from build123d import *

# Parameters (mm, degrees)
ESBO_O1_W                  = 30
ESBO_O1_H                  = 12
RESSALTO_EXTRUS_O1_DEPTH   = 5
CORTE_EXTRUS_O1_DEPTH      = 20.849433241
CORTE_EXTRUS_O1_DEPTH_BACK = 20.849433241
ESBO_O3_R                  = 1.75
CORTE_EXTRUS_O2_DEPTH      = 20
ESBO_O4_R                  = 1.75
CORTE_EXTRUS_O3_DEPTH      = 4
CORTE_EXTRUS_O4_DEPTH      = 20.849433241
CORTE_EXTRUS_O4_DEPTH_BACK = 20.849433241
CHANFRO2_SIZE              = 0.6


with BuildPart() as part:
    # Esboço1 → Ressalto-extrusão1 (new, symmetric)
    with BuildSketch(Plane.XY):
        Rectangle(ESBO_O1_W, ESBO_O1_H)
    extrude(amount=RESSALTO_EXTRUS_O1_DEPTH, both=True)

    # Esboço2 → Corte-extrusão1 (cut, two sides: drawn at the far end of the back side and taken through both)
    with BuildSketch(Plane(origin=(0, 6, 0), x_dir=(1, 0, 0), z_dir=(0, 1, 0)).offset(-CORTE_EXTRUS_O1_DEPTH_BACK)):
        with BuildLine():
            Line((-7.5, 64.244289009), (-7.5, 5))
            ThreePointArc((-7.5, 5), (0, -2.5), (7.5, 5))
            Line((7.5, 5), (7.5, 64.244289009))
            Line((7.5, 64.244289009), (7.5, 182.732867027))
            Line((7.5, 182.732867027), (-7.5, 182.732867027))
            Line((-7.5, 182.732867027), (-7.5, 64.244289009))
        make_face()
    extrude(amount=CORTE_EXTRUS_O1_DEPTH + CORTE_EXTRUS_O1_DEPTH_BACK, mode=Mode.SUBTRACT)

    # Esboço3 → Corte-extrusão2 (cut, through all)
    with BuildSketch(Plane.XY.offset(5)):
        with Locations((11.35, 0)):
            Circle(ESBO_O3_R)
    corte_extrus_o2 = extrude(amount=-CORTE_EXTRUS_O2_DEPTH, mode=Mode.SUBTRACT)

    # Espelhar1: Corte-extrusão2 across plane
    add(corte_extrus_o2.mirror(Plane(origin=(0, 0, 0), x_dir=(0, 0, 1), z_dir=(1, 0, 0))), mode=Mode.SUBTRACT)

    # Esboço4 → Corte-extrusão3 (cut)
    # profile 1 of 2: a face of its own
    with BuildSketch(Plane.XY.offset(5)):
        Polygon((-15, -6), (-8.5, -1.645448267), (-11.35, -3.290896534), (-14.2, -1.645448267), (-14.2, 1.645448267), (-11.35, 3.290896534), (-8.5, 1.645448267), (-15, 6), align=None)
    # profile 2 of 2: a face of its own
    with BuildSketch(Plane.XY.offset(5)):
        Polygon((-11.35, -3.290896534), (-8.5, -1.645448267), (-8.5, 1.645448267), (-11.35, 3.290896534), (-14.2, 1.645448267), (-14.2, -1.645448267), align=None)
        with Locations((-11.35, 0)):
            Circle(ESBO_O4_R, mode=Mode.SUBTRACT)
    corte_extrus_o3 = extrude(amount=-CORTE_EXTRUS_O3_DEPTH, mode=Mode.SUBTRACT)

    # Espelhar2: Corte-extrusão3 across plane
    add(corte_extrus_o3.mirror(Plane(origin=(0, 0, 0), x_dir=(0, 0, 1), z_dir=(1, 0, 0))), mode=Mode.SUBTRACT)

    # Esboço5 → Corte-extrusão4 (cut, two sides: drawn at the far end of the back side and taken through both)
    with BuildSketch(Plane.XZ.offset(6).offset(-CORTE_EXTRUS_O4_DEPTH_BACK)):
        with BuildLine():
            Line((-76.735854523, -34.44642365), (-15, 1))
            ThreePointArc((-15, 1), (0, 5), (15, 1))
            Line((15, 1), (76.735854523, -34.44642365))
            Line((76.735854523, -34.44642365), (76.735854523, 107.930044677))
            Line((76.735854523, 107.930044677), (-76.735854523, 107.930044677))
            Line((-76.735854523, 107.930044677), (-76.735854523, -34.44642365))
        make_face()
    extrude(amount=CORTE_EXTRUS_O4_DEPTH + CORTE_EXTRUS_O4_DEPTH_BACK, mode=Mode.SUBTRACT)

    # Chanfro2
    # the kernel refuses this chamfer: 0.6 mm, written as the material it takes off along each edge
    with BuildSketch(Plane(origin=(-15, 6, -6.543009793), x_dir=(0.9996219169112968, 0.027495876610585904, 0), z_dir=(0, 0, 1)), Plane(origin=(15, 6, 2.543009793), x_dir=(-0.9996219169112968, 0.027495876610585824, 0), z_dir=(0, 0, -1))) as chanfro2_piece_1:
        Polygon((CHANFRO2_SIZE * 0.999621916911, -CHANFRO2_SIZE * 0.0274958766106), (-CHANFRO2_SIZE * 0.0274958766106, -CHANFRO2_SIZE * 0.999621916911), (0, 0), align=None)
    extrude(amount=9.086019586, mode=Mode.SUBTRACT)
    with BuildSketch(Plane(origin=(-16.543009793, 6, -5), x_dir=(0, 0.027495876610585942, 0.9996219169112968), z_dir=(1, 0, 0)), Plane(origin=(5.956990207, 6, -5), x_dir=(0, 0.027495876610585942, 0.9996219169112968), z_dir=(1, 0, 0)), Plane(origin=(16.543009793, -6, -5), x_dir=(0, -0.027495876610585942, 0.9996219169112968), z_dir=(-1, 0, 0)), Plane(origin=(-5.956990207, -6, -5), x_dir=(0, -0.027495876610585942, 0.9996219169112968), z_dir=(-1, 0, 0))) as chanfro2_piece_2:
        Polygon((CHANFRO2_SIZE * 0.999621916911, CHANFRO2_SIZE * 0.0274958766106), (-CHANFRO2_SIZE * 0.0274958766106, CHANFRO2_SIZE * 0.999621916911), (0, 0), align=None)
    extrude(amount=10.586019586, mode=Mode.SUBTRACT)
    with BuildSketch(Plane(origin=(0, 6, -5), x_dir=(0.9788435281484443, 0, -0.20461023288659222), z_dir=(-0.20461023288659222, 0, -0.9788435281484443))) as chanfro2_piece_3:
        Polygon((7.5 + CHANFRO2_SIZE, 0), (7.5, CHANFRO2_SIZE), (7.5, 0), align=None)
    revolve(axis=Axis((0, 6, -5), (0, -1, 0)), revolution_arc=203.613366819, mode=Mode.SUBTRACT)
    with BuildSketch(Plane(origin=(0, 6, -25.125), x_dir=(-0.5416797070080789, 0, 0.8405849719187476), z_dir=(-0.8405849719187476, 0, -0.5416797070080789))) as chanfro2_piece_4:
        Polygon((30.125 - CHANFRO2_SIZE, 0), (30.125, -CHANFRO2_SIZE), (30.125, 0), align=None)
    revolve(axis=Axis((0, 6, -25.125), (0, 1, 0)), revolution_arc=65.596114289, mode=Mode.SUBTRACT)
    with BuildSketch(Plane(origin=(0, -6, -5), x_dir=(0.9788435281484443, 0, -0.20461023288659222), z_dir=(-0.20461023288659222, 0, -0.9788435281484443))) as chanfro2_piece_5:
        Polygon((7.5 + CHANFRO2_SIZE, 0), (7.5, -CHANFRO2_SIZE), (7.5, 0), align=None)
    revolve(axis=Axis((0, -6, -5), (0, -1, 0)), revolution_arc=203.613366819, mode=Mode.SUBTRACT)
    with BuildSketch(Plane(origin=(-15, -6, -6.543009793), x_dir=(0.9996219169112968, -0.027495876610585824, 0), z_dir=(0, 0, 1)), Plane(origin=(15, -6, 2.543009793), x_dir=(-0.9996219169112968, -0.027495876610585904, 0), z_dir=(0, 0, -1))) as chanfro2_piece_6:
        Polygon((CHANFRO2_SIZE * 0.999621916911, CHANFRO2_SIZE * 0.0274958766106), (-CHANFRO2_SIZE * 0.0274958766106, CHANFRO2_SIZE * 0.999621916911), (0, 0), align=None)
    extrude(amount=9.086019586, mode=Mode.SUBTRACT)
    with BuildSketch(Plane(origin=(0, -6, -25.125), x_dir=(-0.5416797070080789, 0, 0.8405849719187476), z_dir=(-0.8405849719187476, 0, -0.5416797070080789))) as chanfro2_piece_7:
        Polygon((30.125, CHANFRO2_SIZE), (30.125 - CHANFRO2_SIZE, 0), (30.125, 0), align=None)
    revolve(axis=Axis((0, -6, -25.125), (0, 1, 0)), revolution_arc=65.596114289, mode=Mode.SUBTRACT)


solid = part.part
Here's how the part is built. I have some questions about the finished solid (model axes, mm). A direction names the side the tool comes from. Coordinates: 2 decimals unless noted, no trailing zeros. Loops run counter-clockwise (first coordinate to the right, second up) from the corner with the lowest first, then second, coordinate; pieces in that order, holes last. Notation, with made-up numbers: (26, 30.25) -> (30, 30.25) arc R34 cw to (30, 66.25) -> close; hole circle Ø8 at (26.5, 25.5). An arc over 180 degrees is marked (long way). Use one line per item in the form item = value. Start each with the question number.
(1) If we section it at B-B (x = 0): Please give me the cut outline in (y, z).
(2) If we section it at D-D (y = 2.75): Please give me the cut outline in (x, z) (3 decimals), then the cut area to 3 significant figures.
(3) We'd pull the mould along Y, two halves only. Please class faces 1 (the face through (-8.5, 0, 2)), 2 (the face through (-0.2, -5.8, 4.6)), 3 (the face through (0, 6, 4)): pulls with the +Y half, pulls with the -Y half, needs draft (parallel to the pull), parting line crosses it, or undercut.
(4) If we section it at C-C (z = -1.75): Give the number of separate pieces and of enclosed holes in the cut face, then the cut area to 3 significant figures.
(5) On a 3-axis mill with a long thin cutter (end or side, diameter ignored), from which of +Z, -Z, +X, -X, +Y, -Y can I reach the whole of each face in a straight line? I mean faces 4 (the face through (14, 0, 1)), 5 (the face through (-10.785, 3.176, 2.099)), 6 (the face through (0.2, 5.6, 2.7)). Say none if no direction works.
(6) If we section it at A-A (y = 0): Please give me the cut outline in (x, z) (3 decimals).
(7) Will these pins go through, and if not, where does the flat tip stop? pin 1 (3.5 mm diameter, centred on x = -12.5, y = -1, fed in from +Z); pin 2 (1.5 mm diameter, centred on y = -1, z = 2.5, fed in from -X); pin 3 (6 mm diameter, centred on y = -4.5, z = 2, fed in from +X); pin 4 (5 mm diameter, centred on x = 10.5, y = 2, fed in from +Z).
(8) Please list where these lines run through material, in increasing order: line 1 along Y through (x, z) = (11.35, -1.2); line 2 along X through (y, z) = (0.5, 0); line 3 along X through (y, z) = (0, -2.7).
Verdict:
q1.outline = (-6, 3.1) -> (-5.4, 2.5) -> (5.4, 2.5) -> (6, 3.1) -> (6, 4.4) -> (5.4, 5) -> (-5.4, 5) -> (-6, 4.4) -> close
q2.outline = (-15, -5) -> (-7.5, -5) arc R7.5 cw to (7.5, -5) -> (15, -5) -> (15, 1) -> (10.149, 1) -> (10.149, 3.239) arc R30.125 ccw to (-10.149, 3.239) -> (-10.149, 1) -> (-15, 1) -> close
q2.area = 161 mm²
q3.face_1 = undercut
q3.face_2 = pulls with the -Y half
q3.face_3 = pulls with the +Y half
q4.separate_pieces = 2
q4.enclosed_holes = 2
q4.area = 177 mm²
q5.face_4 = +Z, +X
q5.face_5 = +Z, -X
q5.face_6 = -Z, +Y
q6.outline = (-15, -5) -> (-13.1, -5) -> (-13.1, 1) -> (-15, 1) -> close; (-9.6, -5) -> (-7.5, -5) arc R7.5 cw to (7.5, -5) -> (9.6, -5) -> (9.6, 1) -> (8.5, 1) -> (8.5, 3.776) arc R30.125 ccw to (-8.5, 3.776) -> (-8.5, 1) -> (-9.6, 1) -> close; (13.1, -5) -> (15, -5) -> (15, 1) -> (13.1, 1) -> close
q7.pin_1 = 1
q7.pin_2 = -8.66
q7.pin_3 = 15
q7.pin_4 = 3.92
q8.line_1 = -6 to -1.75, 1.75 to 6
q8.line_2 = -15 to -13.03, -9.67 to -5.59, 5.59 to 9.67, 13.03 to 15
q8.line_3 = -15 to -13.1, -9.6 to -7.14, 7.14 to 9.6, 13.1 to 15
